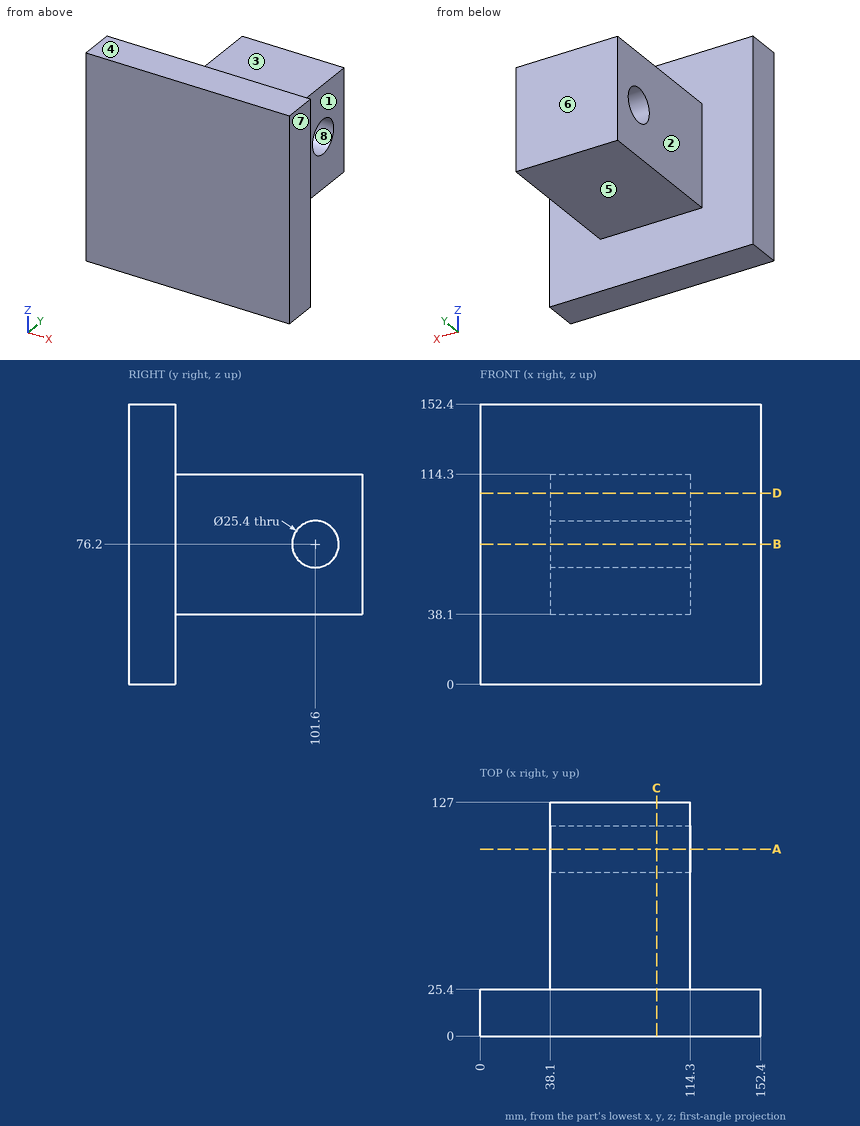
Design review of the part shown in the three views and the two pictorial views. Dimensions are in mm from the part's minimum x, y and z. A direction names the side the tool comes from. Round coordinates to 2 decimals unless told otherwise and drop trailing zeros. Loops run counter-clockwise (first coordinate to the right, second up) from the corner with the lowest first, then second, coordinate; pieces in that order, holes last. Notation, with made-up numbers: M 18,-26.75 L 34,-26.75 A20 cw 34,-9.75 Z; hole C 19.25,63 d10. An arc over 180 degrees is marked long. Answer as a JSON object with one key per item and string values.
Item 1: We need section B-B, the plane z = 76.2. State the section outline as (x, y) points.
Check sheet entries:
{"outline": "M 0,0 L 152.4,0 L 152.4,25.4 L 114.3,25.4 L 114.3,88.9 L 38.1,88.9 L 38.1,25.4 L 0,25.4 Z; M 38.1,114.3 L 114.3,114.3 L 114.3,127 L 38.1,127 Z"}
Item 2: Clearance check with flat-ended pins moving along their axes: P1, Ø4, axis at y = 58.5, z = 87, coming from the -X side; P2, Ø5, axis at x = 102, y = 71, coming from the +Z side; P3, Ø10, axis at x = 48, z = 27, coming from the +Y side. State where each tip first meets the part, or that it passes through.
Check sheet entries:
{"P1": "x = 38.1", "P2": "z = 114.3", "P3": "y = 25.4"}
Item 3: We need section D-D, the plane z = 104. State the section outline as (x, y) points.
Check sheet entries:
{"outline": "M 0,0 L 152.4,0 L 152.4,25.4 L 114.3,25.4 L 114.3,127 L 38.1,127 L 38.1,25.4 L 0,25.4 Z"}
Item 4: We need section A-A, the plane y = 101.6. State the section outline as (x, z) points, and give its area (3 significant figures).
Check sheet entries:
{"outline": "M 38.1,38.1 L 114.3,38.1 L 114.3,63.5 L 38.1,63.5 Z; M 38.1,88.9 L 114.3,88.9 L 114.3,114.3 L 38.1,114.3 Z", "area": "3,870 mm2"}
Item 5: Tool access review of the marked faces 1, 2, 3, 4 and 5: name each direction out of +Z, -Z, +X, -X, +Y, -Y from which nothing blocks a thin tool from reaching the whole face with its end or side.
Check sheet entries:
{"face 1": "+Z, -Z, +X, +Y", "face 2": "+Z, -Z, -X, +Y", "face 3": "+Z, +X, -X, +Y", "face 4": "+Z, +X, -X, +Y, -Y", "face 5": "-Z, +X, -X, +Y"}
Item 6: The part is to be moulded in two halves that separate along Y. For the marked faces 6, 7 and 8, say which applies: +Y half, -Y half, draft (parallel to the pull), parting line (faces both ways), or undercut.
Check sheet entries:
{"face 6": "+Y half", "face 7": "draft", "face 8": "undercut"}
Item 7: We need section C-C, the plane x = 96. State the section outline as (y, z) points, and give its area (3 significant figures).
Check sheet entries:
{"outline": "M 0,0 L 25.4,0 L 25.4,38.1 L 127,38.1 L 127,114.3 L 25.4,114.3 L 25.4,152.4 L 0,152.4 Z; hole C 101.6,76.2 d25.4", "area": "11,100 mm2"}
Item 8: For line 1 along Y through (x, z) = (64, 76.2); line 2 along Z through (x, y) = (65, 101); line 3 along Y through (x, z) = (23, 95), list the stretches that pass through material, from the lowest coordinate up.
Check sheet entries:
{"line 1": "0 to 88.9, 114.3 to 127", "line 2": "38.1 to 63.51, 88.89 to 114.3", "line 3": "0 to 25.4"}
